Part model, mm, in its own coordinate system. A direction names the side the tool comes from. Round coordinates to 2 decimals unless told otherwise and drop trailing zeros. Write each loop counter-clockwise with the first axis right and the second up, starting at its lowest first coordinate (ties: lowest second). Pieces come first, ordered by that corner, then holes. Notation, with made-up numbers: (24, -4.75) -> (55, -4.75) arc R23 ccw to (55, 20.25) -> close; hole circle Ø8 at (48, -27). An arc over 180 degrees is marked (long way). Use CSV: the item, a comma, the result in double quotes. Start each with the question number.
(1) Drop flat-ended pins along their axis: pin 1 (8 mm diameter, centred on x = 26.5, z = 27.5, fed in from -Y); pin 2 (10 mm diameter, centred on y = 26, z = -22, fed in from +X); pin 3 (1.5 mm diameter, centred on y = 22, z = 15.5, fed in from -X); pin 4 (6 mm diameter, centred on x = 8.5, z = 10.5, fed in from -Y). Give the stop position or say it passes through.
(2) Two-plate mould, pull along Z, no slides. Class faces 4 (the flat face through (0, 50.8, -20)), 5 (the cylindrical face through (13.434, -50.685, 13.389)), 6 (the flat face through (-13.36, -0.71, 13.31)): released by +Z, released by -Z, zero draft, split by the parting line, or undercut.
(3) Which spindle directions (+Z, -Z, +X, -X, +Y, -Y) get a long thin tool onto all of the face, cutting with end or side? Do faces 1 (the cylindrical face through (13.389, -50.685, -13.434)), 2 (the flat face through (15.875, -1, 0)), 3 (the cylindrical face through (13.39, 50.69, -13.44)). Say none if no direction does.
(4) Saw through at B-B (z = 0). Give the cut face in (x, y) (1 decimal), plus the area to 3 significant figures.
(5) Saw through at A-A (y = 7). Give the cut face in (x, z) (3 decimals).
(6) Probe line 1 (X direction, y = 1, z = -1) (3 decimals); line 2 (X direction, y = -44.5, z = 10); line 3 (Z direction, x = 12.5, y = 34). List the from-to ranges inside material, lowest first. Write a range as [from, to].
(7) Saw through at C-C (x = 0). Give the cut face in (y, z) (1 decimal).
```python
from build123d import *

# Parameters (mm, degrees)
F0_R     = 38.1
F1_DEPTH = 50.8
F2_R     = 7.9375
F3_W     = 31.75
F3_H     = 31.75
F4_DEPTH = 101.601
F5_SIZE  = 5.08
F6_R     = 3.175
F7_R     = 0.381


with BuildPart() as f1:
    # F0 (on Front) → F1 (new body, symmetric)
    with BuildSketch(Plane.XZ):
        Circle(F0_R)
    extrude(amount=F1_DEPTH, both=True)

    # F2
    f2_edges = [f1.edges().sort_by_distance(p)[0] for p in [
        (-38.1, -50.8, 0),
        (-38.1, 50.8, 0),
    ]]
    fillet(f2_edges, radius=F2_R)

    # F3 (on face) → F4 (cut, through all)
    with BuildSketch(Plane.XZ.offset(50.8)):
        Rectangle(F3_W, F3_H)
    extrude(amount=-F4_DEPTH, mode=Mode.SUBTRACT)

    # F5
    f5_edges = [f1.edges().sort_by_distance(p)[0] for p in [
        (-15.875, 0, 15.875),
        (15.875, 0, -15.875),
        (15.875, 0, 15.875),
        (-15.875, 0, -15.875),
    ]]
    chamfer(f5_edges, length=F5_SIZE)

    # F6
    f6_edges = [f1.edges().sort_by_distance(p)[0] for p in [
        (-10.795, 0, -15.875),
        (-15.875, 0, -10.795),
        (-15.875, 0, 10.795),
        (-10.795, 0, 15.875),
        (10.795, 0, 15.875),
        (15.875, 0, 10.795),
        (15.875, 0, -10.795),
        (10.795, 0, -15.875),
    ]]
    fillet(f6_edges, radius=F6_R)

    # F7
    f7_edges = [f1.edges().sort_by_distance(p)[0] for p in [
        (0, -50.8, 15.875),
        (0, 50.8, 15.875),
    ]]
    fillet(f7_edges, radius=F7_R)


solid = f1.part
```
Answers:
1,pin 1,"stops at y = -49.7"
1,pin 2,"stops at x = 34.1"
1,pin 3,"stops at x = -35.13"
1,pin 4,"passes through"
2,face 4,"zero draft"
2,face 5,"undercut"
2,face 6,"undercut"
3,face 1,"-Y"
3,face 2,"+Y, -Y"
3,face 3,"+Y"
4,outline,"(-38.1, -42.9) arc R7.9 ccw to (-30.2, -50.8) -> (-16.3, -50.8) arc R0.4 ccw to (-15.9, -50.4) -> (-15.9, 50.4) arc R0.4 ccw to (-16.3, 50.8) -> (-30.2, 50.8) arc R7.9 ccw to (-38.1, 42.9) -> close; (15.9, -50.4) arc R0.4 ccw to (16.3, -50.8) -> (30.2, -50.8) arc R7.9 ccw to (38.1, -42.9) -> (38.1, 42.9) arc R7.9 ccw to (30.2, 50.8) -> (16.3, 50.8) arc R0.4 ccw to (15.9, 50.4) -> close"
4,area,"4,460 mm²"
5,outline,"circle Ø76.2 at (0, 0); hole (-15.875, -9.48) arc R3.175 ccw to (-14.945, -11.725) -> (-11.725, -14.945) arc R3.175 ccw to (-9.48, -15.875) -> (9.48, -15.875) arc R3.175 ccw to (11.725, -14.945) -> (14.945, -11.725) arc R3.175 ccw to (15.875, -9.48) -> (15.875, 9.48) arc R3.175 ccw to (14.945, 11.725) -> (11.725, 14.945) arc R3.175 ccw to (9.48, 15.875) -> (-9.48, 15.875) arc R3.175 ccw to (-11.725, 14.945) -> (-14.945, 11.725) arc R3.175 ccw to (-15.875, 9.48) -> close"
6,line 1,"x = [-38.087, -15.875], [15.875, 38.087]"
6,line 2,"x = [-36.59, -15.83], [15.83, 36.59]"
6,line 3,"z = [-35.99, -14.17], [14.17, 35.99]"
7,outline,"(-50.8, -30.2) arc R7.9 ccw to (-42.9, -38.1) -> (42.9, -38.1) arc R7.9 ccw to (50.8, -30.2) -> (50.8, -16.3) arc R0.4 ccw to (50.4, -15.9) -> (-50.4, -15.9) arc R0.4 ccw to (-50.8, -16.3) -> close; (-50.8, 16.3) arc R0.4 ccw to (-50.4, 15.9) -> (50.4, 15.9) arc R0.4 ccw to (50.8, 16.3) -> (50.8, 30.2) arc R7.9 ccw to (42.9, 38.1) -> (-42.9, 38.1) arc R7.9 ccw to (-50.8, 30.2) -> close"
